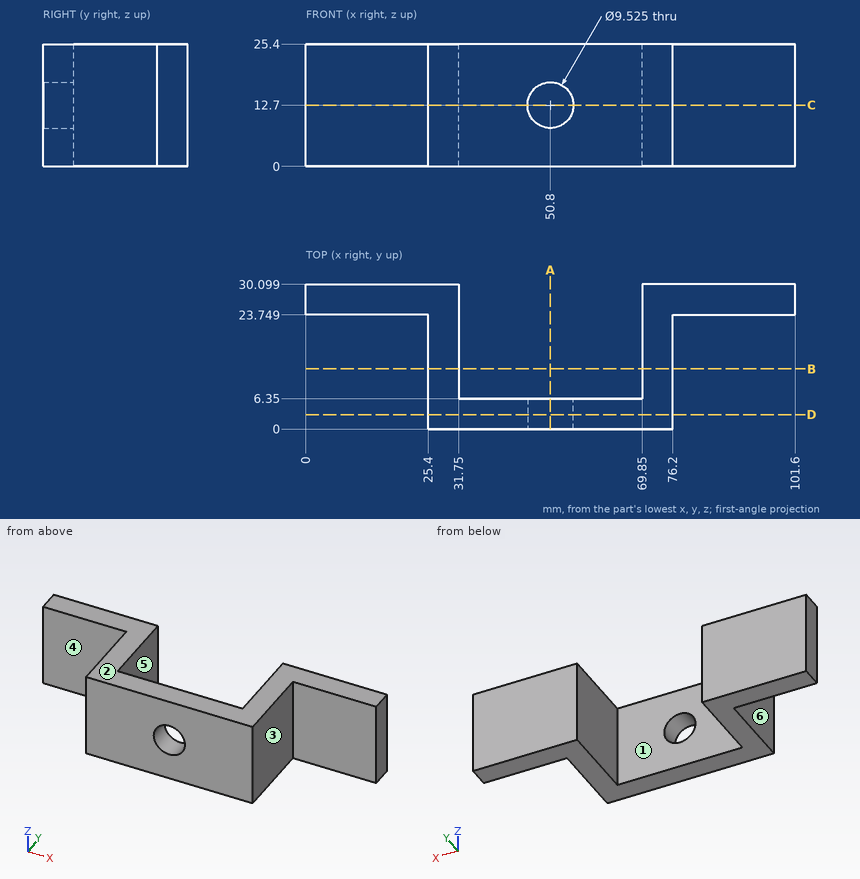
Input: dimensioned drawing with shaded views. Units: mm. Origin: part minimum x, y, z. A direction names the side the tool comes from. Coordinates: 2 decimals unless noted, no trailing zeros. Loops run counter-clockwise (first coordinate to the right, second up) from the corner with the lowest first, then second, coordinate; pieces in that order, holes last. Notation, with made-up numbers: M -9.5,63 L 22.5,63 A17 cw 22.5,85 Z; hole C 51.5,52 d3. An arc over 180 degrees is marked long. Put each result on its own line as item: value.
(1) Draft query along X for the marked faces 4, 5 and 6. Return one class per face: pulls with the +X half, pulls with the -X half, needs draft (parallel to the pull), parting line crosses it, or undercut.
Answer sheet:
face 4: needs draft
face 5: undercut
face 6: pulls with the -X half
(2) Access query for the marked faces 1, 2 and 3. Directions: +Z, -Z, +X, -X, +Y, -Y. A direction counts if a zero-diameter tool reaches every point of the face in a straight line with its end or side. Return the directions, or none.
Answer sheet:
face 1: +Z, -Z, +Y
face 2: +Z, +X, -X, +Y, -Y
face 3: +Z, -Z, +X, -Y
(3) Cut plane D-D on y = 3. Return the cut outline in (x, z) (1 decimal).
Answer sheet:
outline: M 25.4,0 L 76.2,0 L 76.2,25.4 L 25.4,25.4 Z; hole C 50.8,12.7 d9.5
(4) Cut plane C-C on z = 12.7. Return the cut outline in (x, y), then the cut area to 3 significant figures.
Answer sheet:
outline: M 0,23.75 L 25.4,23.75 L 25.4,0 L 46.04,0 L 46.04,6.35 L 31.75,6.35 L 31.75,30.1 L 0,30.1 Z; M 55.56,0 L 76.2,0 L 76.2,23.75 L 101.6,23.75 L 101.6,30.1 L 69.85,30.1 L 69.85,6.35 L 55.56,6.35 Z
area: 886 mm^2
(5) Material intervals for probe 1 along Z at (x, y) = (50.8, 3); probe 2 along X at (y, z) = (14, 10); probe 3 along Y at (x, z) = (7.5, 13.5), sorted ascending.
Answer sheet:
probe 1: z = 0 to 7.94, 17.46 to 25.4
probe 2: x = 25.4 to 31.75, 69.85 to 76.2
probe 3: y = 23.75 to 30.1
(6) First-contact query: pin 1 (12 mm diameter, centred on y = 6.5, z = 15.5, fed in from -X); pin 2 (4 mm diameter, centred on y = 7.5, z = 3, fed in from +X); pin 3 (3 mm diameter, centred on x = 17.5, z = 11, fed in from -Y); pin 4 (7.5 mm diameter, centred on x = 50.8, z = 12.7, fed in from +Y). Flat tips, straight axial feed; report the tip coordinate or a pass-through.
Answer sheet:
pin 1: stops at x = 25.4
pin 2: stops at x = 76.2
pin 3: stops at y = 23.75
pin 4: passes through
(7) Cut plane B-B on y = 12.5. Return the cut outline in (x, z).
Answer sheet:
outline: M 25.4,0 L 31.75,0 L 31.75,25.4 L 25.4,25.4 Z; M 69.85,0 L 76.2,0 L 76.2,25.4 L 69.85,25.4 Z
(8) Cut plane A-A on x = 50.8. Return the cut outline in (y, z), then the cut area to 3 significant figures.
Answer sheet:
outline: M 0,0 L 6.35,0 L 6.35,7.94 L 0,7.94 Z; M 0,17.46 L 6.35,17.46 L 6.35,25.4 L 0,25.4 Z
area: 101 mm^2
